```python
from build123d import *

# Parameters (mm, degrees)
SKETCH1_W           = 22
SKETCH1_H           = 32.6
SKETCH1_W_2         = 14
SKETCH1_H_2         = 24.6
BOSS_EXTRUDE1_DEPTH = 18
SKETCH3_W           = 40
SKETCH3_H           = 40
BOSS_EXTRUDE2_DEPTH = 2
FILLET1_R           = 8


with BuildPart() as part:
    # Sketch1 → Boss-Extrude1 (new body)
    with BuildSketch(Plane(origin=(0, 0, 0), x_dir=(1, 0, 0), z_dir=(0, 1, 0))):
        Rectangle(SKETCH1_W, SKETCH1_H)
        Rectangle(SKETCH1_W_2, SKETCH1_H_2, mode=Mode.SUBTRACT)
    extrude(amount=BOSS_EXTRUDE1_DEPTH)

    # Sketch3 → Boss-Extrude2 (add)
    with BuildSketch(Plane.XZ):
        Rectangle(SKETCH3_W, SKETCH3_H)
    extrude(amount=BOSS_EXTRUDE2_DEPTH)

    # Fillet1
    fillet1_edges = [part.edges().sort_by_distance(p)[0] for p in [
        (20, -1, -20),
        (20, -1, 20),
        (-20, -1, 20),
        (-20, -1, -20),
    ]]
    fillet(fillet1_edges, radius=FILLET1_R)


solid = part.part
```
Work out the finished part from the listing and answer in its coordinate system (mm). A direction names the side the tool comes from. Give positions to 0.01 mm unless a question says otherwise; leave off trailing zeros. Write each loop counter-clockwise with the first axis right and the second up, starting at its lowest first coordinate (ties: lowest second). Pieces come first, ordered by that corner, then holes. Notation, with made-up numbers: (-9.75, 24.25) - (19.25, 24.25) arc R10 cw to (19.25, 29.25) - close; hole circle Ø1 at (-39.75, 0.5). An arc over 180 degrees is marked (long way). Use one line per item in the form item = value.
1. Consider L1, parallel to X at y = 8.5, z = -7; L2, parallel to Y at x = 14.5, z = 11.5; L3, parallel to Z at x = 2, y = 11.5. Determine where each line is inside the solid, lowest interval first.
Filled in:
L1 = -11 to -7, 7 to 11
L2 = -2 to 0
L3 = -16.3 to -12.3, 12.3 to 16.3
2. For faces 1 (the face through (-11, 9, 0)), 2 (the face through (0, 9, 12.3)), 3 (the face through (11, 9, 0)), determine the directions among +Z, -Z, +X, -X, +Y, -Y from which every point of the face is accessible in a straight line to the end or side of a thin tool.
Filled in:
face_1 = +Z, -Z, -X, +Y
face_2 = +Y
face_3 = +Z, -Z, +X, +Y
3. A cutting plane is placed at A-A (y = 8). Write down the section's boundary in (x, z), and give its area (3 significant figures).
Filled in:
outline = (-11, -16.3) - (11, -16.3) - (11, 16.3) - (-11, 16.3) - close; hole (-7, -12.3) - (7, -12.3) - (7, 12.3) - (-7, 12.3) - close
area = 373 mm^2
4. Each of these flat-tipped pins is pushed along its axis until it touches: pin 1 Ø8 at (x, y) = (-10.5, 6) entering from +Z; pin 2 Ø5 at (x, y) = (-4.5, 15.5) entering from -Z; pin 3 Ø4 at (y, z) = (10.5, -5) entering from +X. Where does it stop, or does it pass through?
Filled in:
pin_1 = 16.3
pin_2 = -16.3
pin_3 = 11
5. A cutting plane is placed at C-C (x = -10). Write down the section's boundary in (y, z).
Filled in:
outline = (-2, -20) - (0, -20) - (0, -16.3) - (18, -16.3) - (18, 16.3) - (0, 16.3) - (0, 20) - (-2, 20) - close
6. A cutting plane is placed at B-B (z = 10.5). Write down the section's boundary in (x, y), and give its area (3 significant figures).
Filled in:
outline = (-20, -2) - (20, -2) - (20, 0) - (11, 0) - (11, 18) - (7, 18) - (7, 0) - (-7, 0) - (-7, 18) - (-11, 18) - (-11, 0) - (-20, 0) - close
area = 224 mm^2
7. Determine the mould class of faces 4 (the face through (0, -2, 0)), 5 (the face through (17.594, -1.014, 17.719)), 6 (the face through (0, 0, 0)), 7 (the face through (0, 9, -12.3)) for opening direction Z: released by +Z, released by -Z, zero draft, split by the parting line, or undercut.
Filled in:
face_4 = zero draft
face_5 = released by +Z
face_6 = undercut
face_7 = undercut
8. A cutting plane is placed at D-D (x = -3). Write down the section's boundary in (y, z), and give its area (3 significant figures).
Filled in:
outline = (-2, -20) - (0, -20) - (0, -16.3) - (18, -16.3) - (18, -12.3) - (0, -12.3) - (0, 12.3) - (18, 12.3) - (18, 16.3) - (0, 16.3) - (0, 20) - (-2, 20) - close
area = 224 mm^2
